Verification items for the finished model (mm, model axes). A direction names the side the tool comes from. Give positions to 0.01 mm unless a question says otherwise; leave off trailing zeros. Order: outer loops, then holes, each group sorted by start corner. A loop starts at its lowest first (then second) coordinate and runs counter-clockwise, first axis right, second up.
from build123d import *

# Parameters (mm, degrees)
SKETCH1_W           = 50
SKETCH1_H           = 50
BOSS_EXTRUDE1_DEPTH = 40
SKETCH5_R           = 10.057084534
CUT_EXTRUDE1_DEPTH  = 3
SKETCH4_R           = 10.057084534
CUT_EXTRUDE2_DEPTH  = 3
SKETCH2_R           = 17
CUT_EXTRUDE3_DEPTH  = 3


with BuildPart() as part:
    # Sketch1 → Boss-Extrude1 (new body)
    with BuildSketch(Plane(origin=(0, 0, 0), x_dir=(1, 0, 0), z_dir=(0, 1, 0))):
        Rectangle(SKETCH1_W, SKETCH1_H)
    extrude(amount=BOSS_EXTRUDE1_DEPTH)

    # Sketch5 → Cut-Extrude1 (cut)
    with BuildSketch(Plane(origin=(25, 0, 0), x_dir=(0, 0, -1), z_dir=(1, 0, 0))):
        with Locations((0, 20)):
            Circle(SKETCH5_R)
    extrude(amount=-CUT_EXTRUDE1_DEPTH, mode=Mode.SUBTRACT)

    # Sketch4 → Cut-Extrude2 (cut)
    with BuildSketch(Plane.XY.offset(25)):
        with Locations((0, 20)):
            Circle(SKETCH4_R)
    extrude(amount=-CUT_EXTRUDE2_DEPTH, mode=Mode.SUBTRACT)

    # Sketch2 → Cut-Extrude3 (cut)
    with BuildSketch(Plane.XZ):
        Circle(SKETCH2_R)
    extrude(amount=-CUT_EXTRUDE3_DEPTH, mode=Mode.SUBTRACT)


solid = part.part
(1) Section check B-B, the plane z = 0. Enter the section's corners in (x, y).
Solved:
outline: (-25, 0) - (-17, 0) - (-17, 3) - (17, 3) - (17, 0) - (25, 0) - (25, 9.94) - (22, 9.94) - (22, 30.06) - (25, 30.06) - (25, 40) - (-25, 40) - close
(2) Release check for a two-part mould opening along X. For faces 4 (the flat face through (0, 20, 22)), 5 (the flat face through (-25, 20, 0)), 6 (the flat face through (22, 20, 0)) record: pulls with the +X half, pulls with the -X half, needs draft (parallel to the pull), parting line crosses it, or undercut.
Solved:
face 4: undercut
face 5: pulls with the -X half
face 6: pulls with the +X half
(3) Go/stop test with flat-tipped pins: pin 1 (12 mm diameter, centred on x = -12, z = -14.5, fed in from -Y); pin 2 (6 mm diameter, centred on x = -3, y = 25, fed in from +Z). Record where each tip stops, or that it passes through.
Solved:
pin 1: stops at y = 0
pin 2: stops at z = 22
(4) Section check A-A, the plane y = 20. Enter the section's corners in (x, z).
Solved:
outline: (-25, -25) - (25, -25) - (25, -10.06) - (22, -10.06) - (22, 10.06) - (25, 10.06) - (25, 25) - (10.06, 25) - (10.06, 22) - (-10.06, 22) - (-10.06, 25) - (-25, 25) - close
(5) Section check C-C, the plane x = 11.5. Enter the section's corners in (y, z).
Solved:
outline: (0, -25) - (40, -25) - (40, 25) - (0, 25) - (0, 12.52) - (3, 12.52) - (3, -12.52) - (0, -12.52) - close
(6) Scan lines: line 1 (Y direction, x = 23.3, z = 0); line 2 (Z direction, x = 0, y = 1.9); line 3 (X direction, y = 21, z = -2.5). Record each from-to range of solid material in increasing order.
Solved:
line 1: y = 0 to 9.94, 30.06 to 40
line 2: z = -25 to -17, 17 to 25
line 3: x = -25 to 22
(7) Set-up check for faces 1 (the flat face through (0, 3, 0)), 2 (the cylindrical face through (23.52, 10.18, 2.18)), 3 (the cylindrical face through (-2.18, 10.18, 23.52)): record each of +Z, -Z, +X, -X, +Y, -Y from which the full face is reachable in a straight line by a thin tool's end or side.
Solved:
face 1: -Y
face 2: +X
face 3: +Z
